```python
from build123d import *

# Parameters (mm, degrees)
SKETCH1_R            = 1.3
BOSS_EXTRUDE10_DEPTH = 4
SKETCH1_22_W         = 3
SKETCH1_22_H         = 30
BOSS_EXTRUDE11_DEPTH = 39
FILLET4_R            = 5
SKETCH4_R            = 1.5
SKETCH4_R_2          = 3
CUT_EXTRUDE19_DEPTH  = 126.8173279


with BuildPart() as part:
    # Sketch1 → Boss-Extrude10 (new body)
    with BuildSketch(Plane(origin=(0, 0, 0), x_dir=(1, 0, 0), z_dir=(0, 1, 0))):
        Polygon((0, 70), (0, 50), (3, 50), (3, 20), (0, 20), (0, 0), (100, 0), (100, 70), align=None)
        with Locations(Location((5, 5, 0), (0, 0, 270))):
            Circle(SKETCH1_R, mode=Mode.SUBTRACT)
        with Locations(Location((95, 5, 0), (0, 0, 270))):
            Circle(SKETCH1_R, mode=Mode.SUBTRACT)
        with BuildLine():
            ThreePointArc((15, 16), (11, 20), (15, 24))
            Line((15, 24), (85, 24))
            ThreePointArc((85, 24), (89, 20), (85, 16))
            Line((85, 16), (15, 16))
        make_face(mode=Mode.SUBTRACT)
        with Locations(Location((5, 65, 0), (0, 0, 270))):
            Circle(SKETCH1_R, mode=Mode.SUBTRACT)
        with BuildLine():
            ThreePointArc((15, 31), (11, 35), (15, 39))
            Line((15, 39), (85, 39))
            ThreePointArc((85, 39), (89, 35), (85, 31))
            Line((85, 31), (15, 31))
        make_face(mode=Mode.SUBTRACT)
        with BuildLine():
            ThreePointArc((15, 46), (11, 50), (15, 54))
            Line((15, 54), (85, 54))
            ThreePointArc((85, 54), (89, 50), (85, 46))
            Line((85, 46), (15, 46))
        make_face(mode=Mode.SUBTRACT)
        with Locations(Location((95, 65, 0), (0, 0, 270))):
            Circle(SKETCH1_R, mode=Mode.SUBTRACT)
    extrude(amount=BOSS_EXTRUDE10_DEPTH)

    # Sketch1_22 → Boss-Extrude11 (add)
    with BuildSketch(Plane(origin=(0, 0, 0), x_dir=(1, 0, 0), z_dir=(0, 1, 0))):
        with Locations((1.5, 35)):
            Rectangle(SKETCH1_22_W, SKETCH1_22_H)
    extrude(amount=BOSS_EXTRUDE11_DEPTH)

    # Fillet4
    fillet4_edges = [part.edges().sort_by_distance(p)[0] for p in [
        (1.5, 4, -50),
        (1.5, 39, -20),
        (1.5, 39, -50),
        (1.5, 4, -20),
    ]]
    fillet(fillet4_edges, radius=FILLET4_R)

    # Sketch4 → Cut-Extrude19 (cut, through all)
    with BuildSketch(Plane(origin=(3, 0, 0), x_dir=(0, 0, -1), z_dir=(1, 0, 0))):
        with Locations((26.35, 29)):
            Circle(SKETCH4_R)
        with Locations((43.65, 29)):
            Circle(SKETCH4_R)
        with Locations((35, 8.5)):
            Circle(SKETCH4_R_2)
    extrude(amount=-CUT_EXTRUDE19_DEPTH, mode=Mode.SUBTRACT)

    # Mirror7: part across plane


with BuildPart() as part_1:
    add(part.part)
    add(part.part.mirror(Plane(origin=(50, 0, 0), x_dir=(0, 0, 1), z_dir=(1, 0, 0))))


solid = part_1.part
```
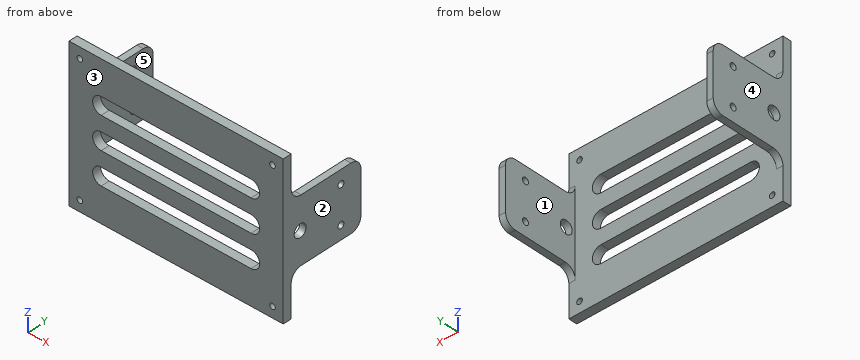
For this review, take the finished solid that the model builds, in its own axes (mm). Face numbers are marked on the shaded views. A direction names the side the tool comes from. Round coordinates to 2 decimals unless told otherwise and drop trailing zeros. Write each loop counter-clockwise with the first axis right and the second up, starting at its lowest first coordinate (ties: lowest second). Pieces come first, ordered by that corner, then holes. Notation, with made-up numbers: (-13.75, 69.5) - (-3.75, 69.5) arc R17 ccw to (-3.75, 83.5) - close; hole circle Ø6 at (75, 19). An arc over 180 degrees is marked (long way). Answer as CSV lines item,"result". Start each with the question number.
(1) For line 1 (Z direction, x = 34, y = 2); line 2 (X direction, y = 2.5, z = -5); line 3 (X direction, y = 17.5, z = -40.5), list the stretches that pass through material, from the lowest coordinate up.
(2) For pin 1 (8 mm diameter, centred on x = 18, z = -57, fed in from +Y); pin 2 (1.5 mm diameter, centred on x = 2, y = 25.5, fed in from +Z), all flat-tipped, find the tip position at first contact; note any pin that passes through.
(3) Add section A-A, the plane y = 15.5. State the section outline as (x, z) points, plus the area to 3 significant figures.
(4) Machinability: for the marked faces 4 and 5, which of the approach directions +Z, -Z, +X, -X, +Y, -Y give a long, thin tool a straight path to every point of the face, cutting with its end or side? Answer none if there is none.
(5) Mouldability with a two-part tool opening along X and no side actions: class the marked faces 1, 2 and 3 as +X half, -X half, draft (parallel to the pull), parting line (faces both ways), or undercut.
(6) Add section C-C, the plane z = -65. State the section outline as (x, y) points, plus the area to 3 significant figures.
(7) Add section B-B, the plane x = 20.5. State the section outline as (y, z) points, plus the area to 3 significant figures.
(8) Add section D-D, the plane x = 95. State the section outline as (y, z) points.
From the geometry:
1,line 1,"z = -70 to -54, -46 to -39, -31 to -24, -16 to 0"
1,line 2,"x = 0 to 3.7, 6.3 to 93.7, 96.3 to 100"
1,line 3,"x = 0 to 3, 97 to 100"
2,pin 1,"stops at y = 4"
2,pin 2,"stops at z = -20"
3,outline,"(0, -50) - (3, -50) - (3, -20) - (0, -20) - close; (97, -50) - (100, -50) - (100, -20) - (97, -20) - close"
3,area,"180 mm²"
4,face 4,"+Z, -Z, -X, +Y, -Y"
4,face 5,"+Z, -Z, +Y"
5,face 1,"undercut"
5,face 2,"+X half"
5,face 3,"draft"
6,outline,"(0, 0) - (3.7, 0) - (3.7, 4) - (0, 4) - close; (6.3, 0) - (93.7, 0) - (93.7, 4) - (6.3, 4) - close; (96.3, 0) - (100, 0) - (100, 4) - (96.3, 4) - close"
6,area,"379 mm²"
7,outline,"(0, -70) - (4, -70) - (4, -54) - (0, -54) - close; (0, -46) - (4, -46) - (4, -39) - (0, -39) - close; (0, -31) - (4, -31) - (4, -24) - (0, -24) - close; (0, -16) - (4, -16) - (4, 0) - (0, 0) - close"
7,area,"184 mm²"
8,outline,"(0, -70) - (4, -70) - (4, -66.3) - (0, -66.3) - close; (0, -63.7) - (4, -63.7) - (4, -6.3) - (0, -6.3) - close; (0, -3.7) - (4, -3.7) - (4, 0) - (0, 0) - close"
